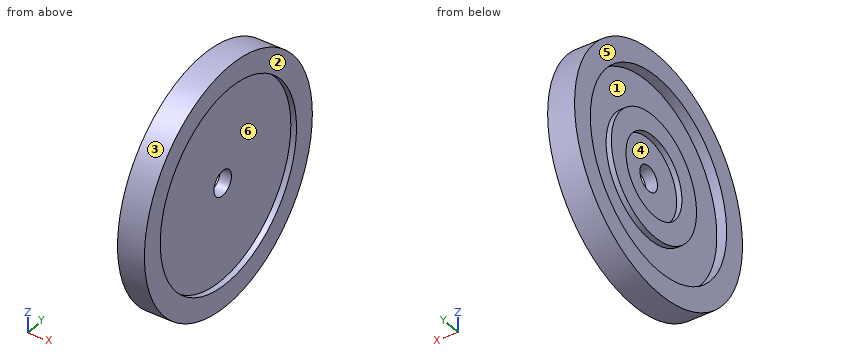
```python
from build123d import *

# Parameters (mm, degrees)
SKETCH2_R           = 17.5
SKETCH2_R_2         = 11.5
BOSS_EXTRUDE1_DEPTH = 1.5
SKETCH4_R           = 3.6
CUT_EXTRUDE2_DEPTH  = 50.033808745


with BuildPart() as part:
    # Sketch1 → Revolve1 (revolve)
    with BuildSketch(Plane.XY):
        Polygon((0, 0), (0, 28), (-2.8, 28), (-2.8, 34.5), (4.88, 34.5), (4.88, 28), (3.25, 28), (3.25, 0), align=None)
    revolve(axis=Axis((3.25, 0, 0), (-1, 0, 0)))

    # Sketch2 → Boss-Extrude1 (add)
    with BuildSketch(Plane.ZY):
        with Locations(Location((0, 0, 0), (0, 0, 270))):
            Circle(SKETCH2_R)
        with Locations(Location((0, 0, 0), (0, 0, 270))):
            Circle(SKETCH2_R_2, mode=Mode.SUBTRACT)
    extrude(amount=BOSS_EXTRUDE1_DEPTH)

    # Sketch4 → Cut-Extrude2 (cut, through all)
    with BuildSketch(Plane(origin=(0, 0, 0), x_dir=(0, 0, -1), z_dir=(1, 0, 0))):
        with Locations(Location((0, 0, 0), (0, 0, 90))):
            Circle(SKETCH4_R)
    extrude(amount=CUT_EXTRUDE2_DEPTH, mode=Mode.SUBTRACT)


solid = part.part
```
CAD build for the part. Positions are in the model's coordinates, mm. Face numbers are marked on the shaded views. A direction names the side the tool comes from. Round coordinates to 2 decimals unless told otherwise and drop trailing zeros. Order: outer loops, then holes, each group sorted by start corner. A loop starts at its lowest first (then second) coordinate and runs counter-clockwise, first axis right, second up. Notation, with made-up numbers: (62, 84.25) - (114, 84.25) arc R27 cw to (114, 120.25) - close; hole circle Ø6 at (33, 7.5). An arc over 180 degrees is marked (long way). Answer in a Markdown table with one row per item. Add a question column.
(1) Probe L1, parallel to Z at x = -0.75, y = 0; L2, parallel to Y at x = 1.95, z = 0; L3, parallel to Z at x = 4.1, y = 0. List the from-to ranges inside material, lowest first. Write a range as [from, to].
(2) Band-saw the part on C-C on x = 1.5. List the corners of the cut face in (y, z), and give its area (3 significant figures).
(3) Drop flat-ended pins along their axis: pin 1 Ø2 at (x, y) = (0.5, -27.5) entering from +Z; pin 2 Ø10.5 at (y, z) = (1, 3.5) entering from -X; pin 3 Ø12 at (y, z) = (-11.5, -13.5) entering from -X. Give the stop position or say it passes through.
(4) Mould opens along Z. For the marked faces 1, 2 and 3 say: +Z half, -Z half, draft (parallel to the pull), parting line (faces both ways), or undercut.
(5) Band-saw the part on A-A on z = 0. List the corners of the cut face in (x, y), and give its area (3 significant figures).
(6) Band-saw the part on D-D on z = -8.5. List the corners of the cut face in (x, y).
(7) 3-axis set-ups, long thin cutter, end or side, ignore diameter. For the marked faces 4, 5 and 6: which of +Z, -Z, +X, -X, +Y, -Y reach the whole face in a straight line?
Data:
| question | item | result |
|---|---|---|
| 1 | L1 | z = [-34.5, -28], [-17.5, -11.5], [11.5, 17.5], [28, 34.5] |
| 1 | L2 | y = [-34.5, -3.6], [3.6, 34.5] |
| 1 | L3 | z = [-34.5, -28], [28, 34.5] |
| 2 | outline | circle Ø69 at (0, 0); hole circle Ø7.2 at (0, 0) |
| 2 | area | 3,700 mm^2 |
| 3 | pin 1 | stops at z = 22.09 |
| 3 | pin 2 | stops at x = 0 |
| 3 | pin 3 | stops at x = -1.5 |
| 4 | face 1 | undercut |
| 4 | face 2 | draft |
| 4 | face 3 | parting line |
| 5 | outline | (-2.8, -34.5) - (4.88, -34.5) - (4.88, -28) - (3.25, -28) - (3.25, -3.6) - (0, -3.6) - (0, -11.5) - (-1.5, -11.5) - (-1.5, -17.5) - (0, -17.5) - (0, -28) - (-2.8, -28) - close; (-2.8, 28) - (0, 28) - (0, 17.5) - (-1.5, 17.5) - (-1.5, 11.5) - (0, 11.5) - (0, 3.6) - (3.25, 3.6) - (3.25, 28) - (4.88, 28) - (4.88, 34.5) - (-2.8, 34.5) - close |
| 5 | area | 276 mm^2 |
| 6 | outline | (-2.8, -33.44) - (4.88, -33.44) - (4.88, -26.68) - (3.25, -26.68) - (3.25, 26.68) - (4.88, 26.68) - (4.88, 33.44) - (-2.8, 33.44) - (-2.8, 26.68) - (0, 26.68) - (0, 15.3) - (-1.5, 15.3) - (-1.5, 7.75) - (0, 7.75) - (0, -7.75) - (-1.5, -7.75) - (-1.5, -15.3) - (0, -15.3) - (0, -26.68) - (-2.8, -26.68) - close |
| 7 | face 4 | -X |
| 7 | face 5 | +Z, -Z, -X, +Y, -Y |
| 7 | face 6 | +X |
